Autodesk Inventor part; units mm, degrees
ref_plane "YZ Plane" through (0, 0, 0) normal (1, 0, 0) x (0, 1, 0)
ref_plane "XZ Plane" through (0, 0, 0) normal (0, 1, 0) x (-1, 0, 0)
ref_plane "XY Plane" through (0, 0, 0) normal (0, 0, 1) x (1, 0, 0)
sketch "Sketch1" plane through (0, 0, 0) normal (0, 1, 0) x (-1, 0, 0)
  circle A0 centre (0, 0) radius 4
  circle A1 centre (0, 0) radius 14
  dimension "d0" = 28
  dimension "d1" = 8
extrude "Extrusion1" add sketch "Sketch1" along normal blind 1
sketch "Sketch2" plane through (0, 1, 0) normal (0, 1, 0) x (1, 0, 0)
  circle A0 centre (0, 0) radius 4
  circle A1 centre (0, 0) radius 12.5
  dimension "d4" = 25
  dimension "d7" = 8
extrude "Extrusion2" add sketch "Sketch2" along normal blind 7
sketch "Sketch3" plane through (0, 8, 0) normal (0, 1, 0) x (1, 0, 0)
  circle A0 centre (0, 0) radius 4
  circle A1 centre (0, 0) radius 14
extrude "Extrusion3" add sketch "Sketch3" along normal blind 1
sketch "Sketch4" plane through (0, 9, 0) normal (0, 1, 0) x (1, 0, 0)
  circle A0 centre (0, 0) radius 4
  circle A1 centre (0, 0) radius 9
  circle A2 centre (0, 0) radius 4
  dimension "d10" = 18
extrude "Extrusion4" add sketch "Sketch4" along normal blind 5.5
properties part number "big_gear"
Could you check a few things on this model? Use its own coordinates, in mm. A direction names the side the tool comes from. Give positions to 0.01 mm unless a question says otherwise; leave off trailing zeros. Write each loop counter-clockwise with the first axis right and the second up, starting at its lowest first coordinate (ties: lowest second). Pieces come first, ordered by that corner, then holes. Notation, with made-up numbers: (4, 64) -> (9, 64) arc R20 cw to (9, 94) -> close; hole circle Ø7 at (42, 5.25). An arc over 180 degrees is marked (long way). Write each question's results on one line, items separated by ' | '. Start each with the question number.
Q1. Which directions (+Z, -Z, +X, -X, +Y, -Y) give clear straight access to the entire face, cutting with the end or side of a thin tool? Please do faces 5 (the face through (11.923, 4.451, 3.755)), 6 (the face through (-1.172, 11.712, 8.923)), 7 (the face through (2, 14.5, 4)).
Q2. I need wall thicknesses on probe 1 along X at (y, z) = (13.4, 0); probe 2 along Y at (x, z) = (-11.5, 7.25). Which ranges of each line are inside material? Lowest first, please.
Q3. We'd pull the mould along Y, two halves only. Please class faces 1 (the face through (12.932, 8.493, -5.362)), 2 (the face through (-5.3, 8, -11.5)), 3 (the face through (5.3, 1, 11.5)), 4 (the face through (9, 9, 3)): +Y half, -Y half, draft (parallel to the pull), parting line (faces both ways), or undercut.
Q4. Suppose I cut it at A-A, the plane z = -3.5. List the corners of the cut face in (x, y) for me, and give its area (3 significant figures).
Q5. I'm going to push flat-ended pins straight in: pin 1 Ø6 at (x, z) = (-4, 9.5) entering from -Y; pin 2 Ø3 at (y, z) = (8.5, -9) entering from -X; pin 3 Ø1.5 at (x, y) = (6.5, 5.5) entering from -Z; pin 4 Ø4 at (x, y) = (-7, 5) entering from -Z. Where does each tip first touch, or does it pass through?
Q6. Suppose I cut it at D-D, the plane y = 4. List the corners of the cut face in (x, z) for me.
Q7. Suppose I cut it at C-C, the plane z = 4.75. List the corners of the cut face in (x, y) for me, and give its area (3 significant figures).
Outcome:
1) face 5: none | face 6: +Y | face 7: +Z, -Z, +X, -X, +Y
2) probe 1: -9 to -4, 4 to 9 | probe 2: 0 to 1, 8 to 9
3) face 1: draft | face 2: undercut | face 3: undercut | face 4: +Y half
4) outline: (-13.56, 0) -> (-1.94, 0) -> (-1.94, 14.5) -> (-8.29, 14.5) -> (-8.29, 9) -> (-13.56, 9) -> (-13.56, 8) -> (-12, 8) -> (-12, 1) -> (-13.56, 1) -> close; (1.94, 0) -> (13.56, 0) -> (13.56, 1) -> (12, 1) -> (12, 8) -> (13.56, 8) -> (13.56, 9) -> (8.29, 9) -> (8.29, 14.5) -> (1.94, 14.5) -> close | area: 257 mm2
5) pin 1: y = 0 | pin 2: x = -11.82 | pin 3: z = -11.1 | pin 4: z = -11.46
6) outline: circle Ø25 at (0, 0); hole circle Ø8 at (0, 0)
7) outline: (-13.17, 0) -> (13.17, 0) -> (13.17, 1) -> (11.56, 1) -> (11.56, 8) -> (13.17, 8) -> (13.17, 9) -> (7.64, 9) -> (7.64, 14.5) -> (-7.64, 14.5) -> (-7.64, 9) -> (-13.17, 9) -> (-13.17, 8) -> (-11.56, 8) -> (-11.56, 1) -> (-13.17, 1) -> close | area: 299 mm2
